from build123d import *

# Parameters (mm, degrees)
F0_W      = 30
F0_H      = 40
F1_DEPTH  = 25.4
F3_W      = 7.5436746702
F3_H      = 13.6774647981
F4_DEPTH  = 25.4
F5_W      = 4.043773748
F5_H      = 10.6986747123
F6_DEPTH  = 12.954
F7_W      = 1.6801413149
F7_H      = 6.6922605038
F8_DEPTH  = 25.4
F9_W      = 21.6371780261
F9_H      = 15.7099463977
F10_DEPTH = 10.922
F11_W     = 8.9419111609
F11_H     = 6.2935836613
F12_DEPTH = 12.6496255398


with BuildPart() as f1:
    # F0 (on Top) → F1 (new body)
    with BuildSketch(Plane.XY):
        with Locations((0.5621314049, -1.8406331738)):
            Rectangle(F0_W, F0_H)
    extrude(amount=F1_DEPTH)

    # F3 (on face) → F4 (join)
    with BuildSketch(Plane.XY.offset(25.4)):
        with Locations((-7.7819279395, -6.838732399)):
            Rectangle(F3_W, F3_H)
    extrude(amount=F4_DEPTH)

    # F5 (on face) → F6 (cut)
    with BuildSketch(Plane.XY.offset(25.4)):
        with Locations((11.5681807511, -8.9288947638)):
            Rectangle(F5_W, F5_H)
    extrude(amount=-F6_DEPTH, mode=Mode.SUBTRACT)

    # F7 (on Right) → F8 (join)
    with BuildSketch(Plane.YZ):
        with Locations((8.8164666668, 3.3461302519)):
            Rectangle(F7_W, F7_H)
    extrude(amount=F8_DEPTH)

    # F9 (on face) → F10 (cut)
    with BuildSketch(Plane(origin=(-14.4378685951, 0, 0), x_dir=(0, -1, 0), z_dir=(-1, 0, 0))):
        with Locations((-4.5737433247, 14.6038669627)):
            Rectangle(F9_W, F9_H)
    extrude(amount=-F10_DEPTH, mode=Mode.SUBTRACT)

    # F11 (on face) → F12 (join)
    with BuildSketch(Plane.YZ.offset(15.5621314049)):
        with Locations((-4.4709555805, 17.0851889998)):
            Rectangle(F11_W, F11_H)
    extrude(amount=F12_DEPTH)


solid = f1.part
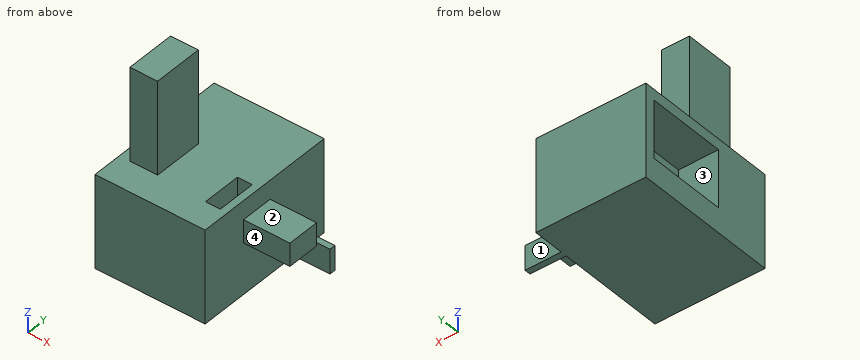
The listing builds one solid part. Answer for the finished solid, in the listing's coordinates (mm). Face numbers are marked on the shaded views. A direction names the side the tool comes from. Round coordinates to 2 decimals unless told otherwise and drop trailing zeros. Write each loop counter-clockwise with the first axis right and the second up, starting at its lowest first coordinate (ties: lowest second). Pieces come first, ordered by that corner, then holes. Notation, with made-up numbers: (45.5, 72.25) - (100.5, 72.25) arc R15 cw to (100.5, 96.25) - close; hole circle Ø6 at (61.25, 30). An arc over 180 degrees is marked (long way). Use a Markdown table: item, result. Add a question column.
1. The part is cut by section A-A (z = 24.5). Write down the section's boundary in (x, y).
2. The part is cut by section B-B (x = 18). Write down the section's boundary in (y, z), and give its area (3 significant figures).
3. Consider line 1 (Y direction, x = -6, z = 8.5); line 2 (X direction, y = -4.5, z = 16.5); line 3 (Z direction, x = -10.5, y = 8). Determine where each line is inside the solid, lowest interval first.
4. Flat-ended cylindrical pins translate along their axes: P1, Ø6, axis at x = 2, y = -12, coming from the +Z side; P2, Ø12, axis at x = -11.5, y = 2, coming from the -Z side; P3, Ø4, axis at x = -7, z = 30, coming from the -Y side; P4, Ø6, axis at y = 7, z = 22.5, coming from the +X side. Find the tip coordinate at first contact, or state that the pin passes through.
5. The part is cut by section C-C (y = -2.5). Write down the section's boundary in (x, z), and give its area (3 significant figures).
6. The part is cut by section D-D (z = 8.5). Write down the section's boundary in (x, y).
7. A tool of negligible diameter and unlimited length cuts with its end or side. For the marked faces 1, 2, 3 and 4, from which of +Z, -Z, +X, -X, +Y, -Y can it reach the whole face along a straight path? Write none if from no direction.
Reported:
| question | item | result |
|---|---|---|
| 1 | outline | (-14.44, -21.84) - (15.56, -21.84) - (15.56, 18.16) - (-14.44, 18.16) - close; hole (9.55, -14.28) - (13.59, -14.28) - (13.59, -3.58) - (9.55, -3.58) - close |
| 2 | outline | (-8.94, 13.94) - (0, 13.94) - (0, 20.23) - (-8.94, 20.23) - close; (7.98, 0) - (9.66, 0) - (9.66, 6.69) - (7.98, 6.69) - close |
| 2 | area | 67.5 mm^2 |
| 3 | line 1 | -21.84 to -6.24, 15.39 to 18.16 |
| 3 | line 2 | -3.52 to 9.55, 13.59 to 28.21 |
| 3 | line 3 | 0 to 6.75, 22.46 to 25.4 |
| 4 | P1 | z = 25.4 |
| 4 | P2 | z = 0 |
| 4 | P3 | y = -13.68 |
| 4 | P4 | x = 15.56 |
| 5 | outline | (-14.44, 0) - (15.56, 0) - (15.56, 13.94) - (28.21, 13.94) - (28.21, 20.23) - (15.56, 20.23) - (15.56, 25.4) - (-4.01, 25.4) - (-4.01, 50.8) - (-11.55, 50.8) - (-11.55, 25.4) - (-14.44, 25.4) - (-14.44, 22.46) - (-3.52, 22.46) - (-3.52, 6.75) - (-14.44, 6.75) - close |
| 5 | area | 862 mm^2 |
| 6 | outline | (-14.44, -21.84) - (15.56, -21.84) - (15.56, 18.16) - (-14.44, 18.16) - (-14.44, 15.39) - (-3.52, 15.39) - (-3.52, -6.24) - (-14.44, -6.24) - close |
| 7 | face 1 | +Z, -Z, +X, +Y |
| 7 | face 2 | +Z, +X, +Y, -Y |
| 7 | face 3 | -X |
| 7 | face 4 | +Z, -Z, +X, -Y |
